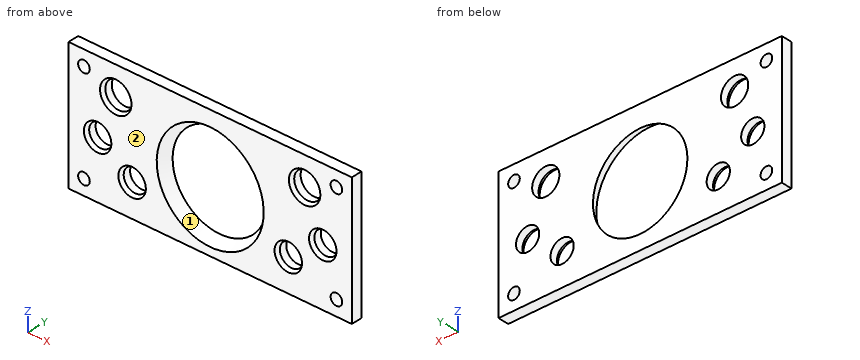
```python
from build123d import *
from OCP.BRepFilletAPI import BRepFilletAPI_MakeChamfer

# Parameters (mm, degrees)
SKETCH1_W           = 78
SKETCH1_H           = 36
SKETCH1_R           = 13
SKETCH1_R_2         = 3.2
SKETCH1_R_3         = 3.75
BOSS_EXTRUDE1_DEPTH = 3
CHAMFER1_SIZE2      = 1.732050808
CHAMFER1_SIZE       = 3
CHAMFER2_SIZE       = 1
CHAMFER2_SIZE2      = 0.577350269
SKETCH2_R           = 1.6
CUT_EXTRUDE1_DEPTH  = 44.058100283


with BuildPart() as part:
    # Sketch1 → Boss-Extrude1 (new body)
    with BuildSketch(Plane(origin=(0, 0, 0), x_dir=(1, 0, 0), z_dir=(0, 1, 0))):
        Rectangle(SKETCH1_W, SKETCH1_H)
        with Locations(Location((0, 1, 0), (0, 0, 270))):
            Circle(SKETCH1_R, mode=Mode.SUBTRACT)
        with Locations(Location((-31, 2, 0), (0, 0, 270))):
            Circle(SKETCH1_R_2, mode=Mode.SUBTRACT)
        with Locations(Location((-26, -10, 0), (0, 0, 270))):
            Circle(SKETCH1_R_3, mode=Mode.SUBTRACT)
        with Locations(Location((31, 2, 0), (0, 0, 270))):
            Circle(SKETCH1_R_2, mode=Mode.SUBTRACT)
        with Locations(Location((26, -10, 0), (0, 0, 270))):
            Circle(SKETCH1_R_3, mode=Mode.SUBTRACT)
        with Locations(Location((21.5, 9, 0), (0, 0, 270))):
            Circle(SKETCH1_R_2, mode=Mode.SUBTRACT)
        with Locations(Location((-21.5, 9, 0), (0, 0, 270))):
            Circle(SKETCH1_R_2, mode=Mode.SUBTRACT)
    extrude(amount=BOSS_EXTRUDE1_DEPTH)

    # Chamfer1
    chamfer1_edges = [part.edges().sort_by_distance(p)[0] for p in [
        (0, 0, -14),
    ]]
    chamfer1_side = [part.faces().sort_by_distance(p)[0] for p in [
        (0, 0.034641016, -14),
    ]]
    chamfer(chamfer1_edges, length=CHAMFER1_SIZE - 0.0001, length2=CHAMFER1_SIZE2 - 0.0001, reference=chamfer1_side[0])  # a hair under: the kernel refuses the full size

    # Chamfer2: one chamfer whose edges measure the first distance from different faces: ONE call of the kernel's chamfer builder (chamfer() names one face for all edges)
    chamfer2_edges_1 = [part.edges().sort_by_distance(p)[0] for p in [
        (-31, 0, -5.2),
    ]]
    chamfer2_side_1 = [part.faces().sort_by_distance(p)[0] for p in [
        (-31, 1.5, -5.2),
    ]]
    chamfer2_edges_2 = [part.edges().sort_by_distance(p)[0] for p in [
        (-26, 0, 6.25),
    ]]
    chamfer2_side_2 = [part.faces().sort_by_distance(p)[0] for p in [
        (-26, 1.5, 6.25),
    ]]
    chamfer2_edges_3 = [part.edges().sort_by_distance(p)[0] for p in [
        (31, 0, -5.2),
    ]]
    chamfer2_side_3 = [part.faces().sort_by_distance(p)[0] for p in [
        (31, 1.5, -5.2),
    ]]
    chamfer2_edges_4 = [part.edges().sort_by_distance(p)[0] for p in [
        (26, 0, 6.25),
    ]]
    chamfer2_side_4 = [part.faces().sort_by_distance(p)[0] for p in [
        (26, 1.5, 6.25),
    ]]
    chamfer2_edges_5 = [part.edges().sort_by_distance(p)[0] for p in [
        (21.5, 0, -12.2),
    ]]
    chamfer2_side_5 = [part.faces().sort_by_distance(p)[0] for p in [
        (21.5, 1.5, -12.2),
    ]]
    chamfer2_edges_6 = [part.edges().sort_by_distance(p)[0] for p in [
        (-21.5, 0, -12.2),
    ]]
    chamfer2_side_6 = [part.faces().sort_by_distance(p)[0] for p in [
        (-21.5, 1.5, -12.2),
    ]]
    chamfer2 = BRepFilletAPI_MakeChamfer(part.part.solid().wrapped)
    for e in chamfer2_edges_1:
        chamfer2.Add(CHAMFER2_SIZE, CHAMFER2_SIZE2, e.wrapped, chamfer2_side_1[0].wrapped)  # the first distance lies on this face
    for e in chamfer2_edges_2:
        chamfer2.Add(CHAMFER2_SIZE, CHAMFER2_SIZE2, e.wrapped, chamfer2_side_2[0].wrapped)  # the first distance lies on this face
    for e in chamfer2_edges_3:
        chamfer2.Add(CHAMFER2_SIZE, CHAMFER2_SIZE2, e.wrapped, chamfer2_side_3[0].wrapped)  # the first distance lies on this face
    for e in chamfer2_edges_4:
        chamfer2.Add(CHAMFER2_SIZE, CHAMFER2_SIZE2, e.wrapped, chamfer2_side_4[0].wrapped)  # the first distance lies on this face
    for e in chamfer2_edges_5:
        chamfer2.Add(CHAMFER2_SIZE, CHAMFER2_SIZE2, e.wrapped, chamfer2_side_5[0].wrapped)  # the first distance lies on this face
    for e in chamfer2_edges_6:
        chamfer2.Add(CHAMFER2_SIZE, CHAMFER2_SIZE2, e.wrapped, chamfer2_side_6[0].wrapped)  # the first distance lies on this face
    add(Compound.cast(chamfer2.Shape()), mode=Mode.REPLACE)

    # Sketch2 → Cut-Extrude1 (cut, through all)
    with BuildSketch(Plane(origin=(0, 3, 0), x_dir=(1, 0, 0), z_dir=(0, 1, 0))):
        with Locations(Location((-34.757359313, -13.757359313, 0), (0, 0, 270))):
            Circle(SKETCH2_R)
        with Locations(Location((-34.757359313, 13.757359313, 0), (0, 0, 270))):
            Circle(SKETCH2_R)
        with Locations(Location((34.757359313, 13.757359313, 0), (0, 0, 270))):
            Circle(SKETCH2_R)
        with Locations(Location((34.757359313, -13.757359313, 0), (0, 0, 270))):
            Circle(SKETCH2_R)
    extrude(amount=-CUT_EXTRUDE1_DEPTH, mode=Mode.SUBTRACT)


solid = part.part
```
Model file for the job. Use its own axes, mm. Face numbers are marked on the shaded views. Round coordinates to 2 decimals unless told otherwise and drop trailing zeros. Order: outer loops, then holes, each group sorted by start corner. A loop starts at its lowest first (then second) coordinate and runs counter-clockwise, first axis right, second up. Notation, with made-up numbers: (16, -23) -> (25, -23) arc R22 cw to (25, 15) -> close; hole circle Ø3 at (-4.5, 54.5). An arc over 180 degrees is marked (long way). Use one line per item in the form item = value.
Item 1: Cut at B-B, the plane y = 1.95. Give the number of separate pieces and of enclosed holes in the cut face, and give its area (3 significant figures).
Returned:
separate_pieces = 1
enclosed_holes = 11
area = 1,980 mm^2
Item 2: Cut at A-A, the plane x = -26. Write the cut outline in (y, z), and give its area (3 significant figures).
Returned:
outline = (0, -18) -> (3, -18) -> (3, 6.25) -> (1, 6.25) -> (0, 5.67) -> close; (0, 14.33) -> (1, 13.75) -> (3, 13.75) -> (3, 18) -> (0, 18) -> close
area = 84.9 mm^2
Item 3: Drill centre lines: line 1 (X direction, y = 1.25, z = -4); line 2 (X direction, y = 0.6, z = 11); line 3 (Z direction, x = -29, y = 1.55). Where is each one in solid material? Low to high.
Returned:
line_1 = -39 to -33.5, -28.5 to -13.69, 13.69 to 28.5, 33.5 to 39
line_2 = -39 to -29.85, -22.15 to -7.93, 7.93 to 22.15, 29.85 to 39
line_3 = -18 to -4.5, 0.5 to 7.75, 12.25 to 18
Item 4: Flat gauge pin, fed straight in: pin 1 Ø4 at (x, z) = (-21.5, -9) entering from -Y. Where does the tip first touch, or does it go through?
Returned:
pin_1 = through
Item 5: Pull direction Z, two halves, no side cores. Call the marked faces 1 and 2: released by +Z, released by -Z, zero draft, split by the parting line, or undercut.
Returned:
face_1 = undercut
face_2 = zero draft
